Check sheet for the modelled part. Datum: model origin and axes. Units: mm. Coordinates: 2 decimals unless noted, no trailing zeros. Loops run counter-clockwise (first coordinate to the right, second up) from the corner with the lowest first, then second, coordinate; pieces in that order, holes last.
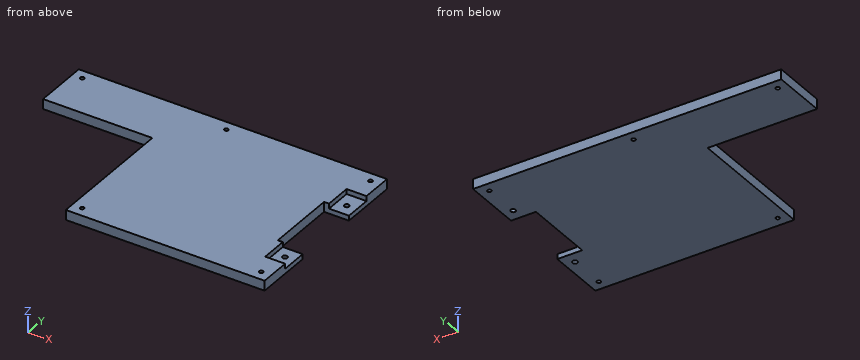
Autodesk Inventor part; units mm, degrees
ref_plane "YZ Plane" through (0, 0, 0) normal (1, 0, 0) x (0, 1, 0)
ref_plane "XZ Plane" through (0, 0, 0) normal (0, 1, 0) x (-1, 0, 0)
ref_plane "XY Plane" through (0, 0, 0) normal (0, 0, 1) x (1, 0, 0)
sketch "Sketch1" plane through (0, 0, 0) normal (0, 0, 1) x (1, 0, 0)
  line L0 (0, 0) -> (620, 0)
  line L1 (110, -188) -> (510, -188)
  line L2 (510, -188) -> (510, -55)
  line L3 (510, -55) -> (620, -55)
  line L4 (620, -55) -> (620, 0)
  line L5 (110, -188) -> (110, -55)
  line L6 (0, -55) -> (0, 0)
  line L7 (0, -55) -> (110, -55)
  point P0 (310, -188)
  point P1 (310, 0)
  dimension "d0" = 620
  dimension "d1" = 188
  dimension "d2" = 400
  dimension "d3" = 133
extrude "Extrusion1" add sketch "Sketch1" along normal blind 10
sketch "Sketch2" plane through (0, 0, 10) normal (0, 0, 1) x (1, 0, 0)
  line L0 (620, 0) -> (0, 0)
  line L1 (510, -188) -> (110, -188)
  line L2 (620, 0) -> (310, 0)
  line L3 (310, 0) -> (310, -188)
  line L4 (310, -188) -> (620, -188)
  line L5 (620, -188) -> (620, 0)
extrude "Extrusion2" cut sketch "Sketch2" against normal through all
sketch "Sketch3" plane through (0, 0, 10) normal (0, 0, 1) x (1, 0, 0)
  circle A0 centre (10, -10) radius 2
  line L0 (310, 0) -> (0, 0)
  line L1 (0, 0) -> (0, -55)
  circle A1 centre (155, -10) radius 2
  circle A2 centre (300, -10) radius 2
  line L2 (310, -188) -> (310, 0)
  line L3 (10, -10) -> (300, -10) construction
  circle A3 centre (120, -178) radius 2
  line L4 (110, -55) -> (110, -188)
  line L5 (110, -188) -> (310, -188)
  circle A4 centre (300, -178) radius 2
  dimension "d8" = 4
  dimension "d9" = 10
  dimension "d10" = 10
  dimension "d11" = 4
  dimension "d12" = 4
  dimension "d13" = 10
  dimension "d14" = 4
  dimension "d15" = 10
  dimension "d16" = 10
  dimension "d17" = 4
  dimension "d18" = 10
  dimension "d19" = 10
extrude "Extrusion3" cut sketch "Sketch3" against normal through all
sketch "Sketch6" plane through (0, 0, 10) normal (0, 0, 1) x (1, 0, 0)
  line L0 (310, -31.5) -> (290, -31.5)
  line L1 (290, -31.5) -> (290, -156.5)
  line L2 (290, -156.5) -> (310, -156.5)
  line L3 (310, -156.5) -> (310, -31.5)
  line L4 (310, -188) -> (310, 0)
  point P0 (0, 0)
  point P1 (310, -94)
  dimension "d42" = 20
  dimension "d43" = 125
extrude "Extrusion6" cut sketch "Sketch6" against normal blind 5
sketch "Sketch7" plane through (0, 0, 5) normal (0, 0, 1) x (1, 0, 0)
  line L0 (300, -46.5) -> (300, -141.5) construction
  circle A0 centre (300, -46.5) radius 2.5
  circle A1 centre (300, -141.5) radius 2.5
  line L1 (310, -31.5) -> (310, -156.5)
  point P0 (0, 0)
  point P1 (300, -94)
  point P2 (310, -94)
  dimension "d46" = 5
  dimension "d47" = 5
  dimension "d48" = 10
  dimension "d49" = 95
extrude "Extrusion7" cut sketch "Sketch7" against normal through all
sketch "Sketch8" plane through (0, 0, 0) normal (0, 0, -1) x (-1, 0, 0)
  line L0 (-285, -58.5) -> (-335, -58.5)
  line L1 (-335, -58.5) -> (-335, -129.5)
  line L2 (-335, -129.5) -> (-285, -129.5)
  line L3 (-285, -129.5) -> (-285, -58.5)
  line L4 (-310, 0) -> (-310, -188)
  point P0 (0, 0)
  point P1 (-335, -94)
  point P2 (-310, -94)
  point P3 (-310, -58.5)
  dimension "d52" = 50
  dimension "d53" = 71
extrude "Extrusion8" cut sketch "Sketch8" against normal through all
properties part number "SP001b" material "ABS Plastic"
(1) Section check C-C, the plane y = -87. Enter the section's corners in (x, z).
(2) Section check B-B, the plane x = 89. Enter the section's corners in (y, z).
(3) Section check A-A, the plane z = 2.5. Enter the section's corners in (x, y), plus the area to 3 significant figures.
(4) Scan lines: line 1 along X through (y, z) = (-178, 4.5); line 2 along Y through (x, z) = (300, 1.7); line 3 along Y through (x, z) = (291, 8.5). Record each from-to range of solid material in increasing order.
(5) Gauge pin test, flat ends, axial feed: P1, Ø6, axis at x = 295.5, y = -44, coming from the +Z side; P2, Ø3.5, axis at x = 300, y = -10, coming from the -Z side; P3, Ø5.5, axis at y = -145.5, z = 8.5, coming from the +X side; P4, Ø5, axis at y = -91.5, z = 5, coming from the +X side. Record the tip position at first contact, or that the pin passes through.
Determined:
1. outline: (110, 0) - (285, 0) - (285, 10) - (110, 10) - close
2. outline: (-55, 0) - (0, 0) - (0, 10) - (-55, 10) - close
3. outline: (0, -55) - (110, -55) - (110, -188) - (310, -188) - (310, -129.5) - (285, -129.5) - (285, -58.5) - (310, -58.5) - (310, 0) - (0, 0) - close; hole circle Ø4 at (10, -10); hole circle Ø4 at (120, -178); hole circle Ø4 at (155, -10); hole circle Ø5 at (300, -141.5); hole circle Ø5 at (300, -46.5); hole circle Ø4 at (300, -178); hole circle Ø4 at (300, -10)
3. area: 41,800 mm2
4. line 1: x = 110 to 118, 122 to 298, 302 to 310
4. line 2: y = -188 to -180, -176 to -144, -139 to -129.5, -58.5 to -49, -44 to -12, -8 to 0
4. line 3: y = -188 to -156.5, -31.5 to 0
5. P1: stops at z = 5
5. P2: passes through
5. P3: stops at x = 290
5. P4: stops at x = 285
